```python
from build123d import *

# Parameters (mm, degrees)
SKETCH1_R           = 16
BOSS_EXTRUDE1_DEPTH = 450
SKETCH2_W           = 65
SKETCH2_H           = 130
BOSS_EXTRUDE2_DEPTH = 65
SKETCH3_R           = 40
BOSS_EXTRUDE3_DEPTH = 10
DOME1_FACE_RADIUS   = 40
DOME1_HEIGHT        = 60


with BuildPart() as part:
    # Sketch1 → Boss-Extrude1 (new body)
    with BuildSketch(Plane(origin=(0, 0, 0), x_dir=(1, 0, 0), z_dir=(0, 1, 0))):
        with Locations(Location((0, 0, 0), (0, 0, 270))):
            Circle(SKETCH1_R)
    extrude(amount=BOSS_EXTRUDE1_DEPTH)

    # Sketch2 → Boss-Extrude2 (add)
    with BuildSketch(Plane(origin=(0, 450, 0), x_dir=(1, 0, 0), z_dir=(0, 1, 0))):
        with Locations((0, 5)):
            Rectangle(SKETCH2_W, SKETCH2_H)
    extrude(amount=BOSS_EXTRUDE2_DEPTH)

    # Sketch3 → Boss-Extrude3 (add)
    with BuildSketch(Plane.XY.offset(60)):
        with Locations(Location((0, 482.5, 0), (0, 0, 144.340912304))):
            Circle(SKETCH3_R)
    extrude(amount=BOSS_EXTRUDE3_DEPTH)

    # Dome1: an elliptical dome of height H over a round flat face of radius A is half a spheroid: the quarter ellipse of half axes A and H revolved about the face's axis
    with BuildSketch(Plane((0, 482.5, 70), x_dir=(0, 1, 0), z_dir=(1, 0, 0)), mode=Mode.PRIVATE) as dome1_quarter:
        Ellipse(DOME1_FACE_RADIUS, DOME1_HEIGHT)
        Rectangle(DOME1_FACE_RADIUS, DOME1_HEIGHT, align=(Align.MIN, Align.MIN), mode=Mode.INTERSECT)
    revolve(dome1_quarter.sketch, axis=Axis((0, 482.5, 70), (0, 0, 1)))


solid = part.part
```
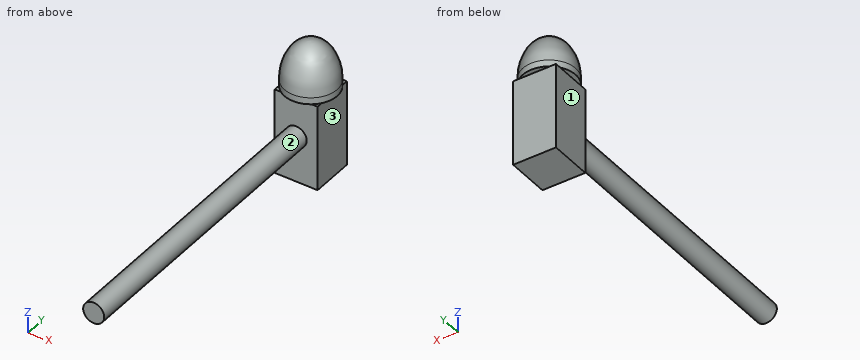
Here's how the part is built. I have some questions about the finished solid (model axes, mm). Face numbers are marked on the shaded views. A direction names the side the tool comes from. Coordinates: 2 decimals unless noted, no trailing zeros. Order: outer loops, then holes, each group sorted by start corner. A loop starts at its lowest first (then second) coordinate and runs counter-clockwise, first axis right, second up. Notation, with made-up numbers: (26, 75.25) - (42, 75.25) arc R23 ccw to (42, 86.25) - close; hole circle Ø7 at (77, 63.5). An arc over 180 degrees is marked (long way). One line per question, with ' | ' between items.
(1) Suppose I cut it at B-B on y = 345. List the corners of the cut face in (x, z) for me.
Report:
outline: circle Ø32 at (0, 0)
(2) Suppose I cut it at A-A on z = 0. List the corners of the cut face in (x, y) for me, and give its area (3 significant figures).
Report:
outline: (-32.5, 450) - (-16, 450) - (-16, 0) - (16, 0) - (16, 450) - (32.5, 450) - (32.5, 515) - (-32.5, 515) - close | area: 18,600 mm2
(3) For the marked faces 1, 2 and 3, which set-ups out of +Z, -Z, +X, -X, +Y, -Y let a thin tool reach every point of the face, with its end or its side?
Report:
face 1: -Z, -X, +Y, -Y | face 2: -Y | face 3: -Z, +X, +Y, -Y
(4) If I drill on L1, parallel to Y at x = 20, z = 59; L2, parallel to X at y = 462.5, z = -15.5; L3, parallel to Y at x = -4, z = 4.5, over which ranges is the centre line in solid material (lowest first)?
Report:
L1: y = 450 to 515 | L2: x = -32.5 to 32.5 | L3: y = 0 to 515
(5) Suppose I cut it at C-C on z = 25. List the corners of the cut face in (x, y) for me, and give its area (4 significant figures).
Report:
outline: (-32.5, 450) - (32.5, 450) - (32.5, 515) - (-32.5, 515) - close | area: 4,225 mm2
(6) Will these pins go through, and if not, where does the flat tip stop? pin 1 (12 mm diameter, centred on y = 380, z = 8, fed in from -X); pin 2 (10 mm diameter, centred on x = 16.5, y = 425.5, fed in from +Z); pin 3 (4 mm diameter, centred on x = -37, y = 479, fed in from -Z).
Report:
pin 1: stops at x = -15.87 | pin 2: stops at z = 11.12 | pin 3: stops at z = 60
